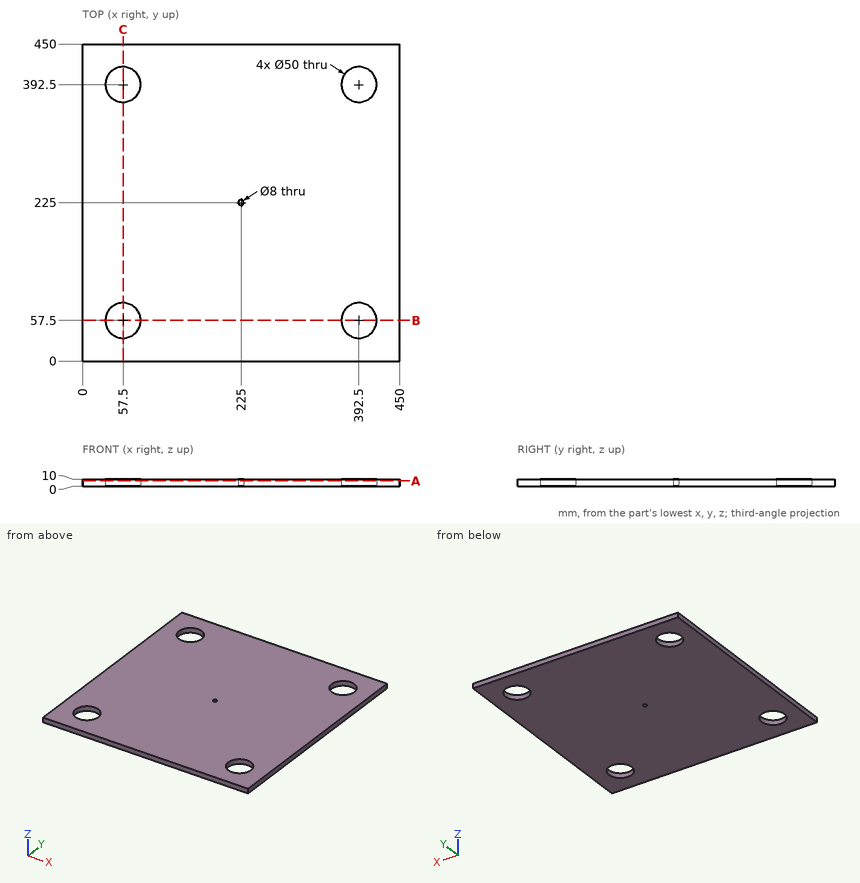
Verification items for this drawing (mm, ordinates from the low corner). Coordinates: 2 decimals unless noted, no trailing zeros. Order: outer loops, then holes, each group sorted by start corner. A loop starts at its lowest first (then second) coordinate and runs counter-clockwise, first axis right, second up. Notation, with made-up numbers: M 23.25,38.25 L 56.25,38.25 A16 cw 56.25,45.25 Z; hole C 8,88.25 d3. An arc over 180 degrees is marked long. Answer as a JSON object with one key per item and string values.
Q1. Cross-section at B-B on y = 57.5. Record the cut outline in (x, z).
Results are:
{"outline": "M 0,0 L 32.5,0 L 32.5,10 L 0,10 Z; M 82.5,0 L 367.5,0 L 367.5,10 L 82.5,10 Z; M 417.5,0 L 450,0 L 450,10 L 417.5,10 Z"}
Q2. Cross-section at A-A on z = 7.25. Record the cut outline in (x, y).
Results are:
{"outline": "M 0,0 L 450,0 L 450,450 L 0,450 Z; hole C 57.5,57.5 d50; hole C 57.5,392.5 d50; hole C 225,225 d8; hole C 392.5,57.5 d50; hole C 392.5,392.5 d50"}
Q3. Scan lines: line 1 (Y direction, x = 392.5, z = 6.75); line 2 (Y direction, x = 225, z = 5); line 3 (X direction, y = 79, z = 3.75). Record each from-to range of solid material in increasing order.
Results are:
{"line 1": "y = 0 to 32.5, 82.5 to 367.5, 417.5 to 450", "line 2": "y = 0 to 221, 229 to 450", "line 3": "x = 0 to 44.74, 70.26 to 379.74, 405.26 to 450"}
